```python
from build123d import *

# Parameters (mm, degrees)
SKETCH1_R           = 2.5
BOSS_EXTRUDE1_DEPTH = 9
FILLET1_R           = 0.3
SKETCH2_W           = 3
SKETCH2_H           = 3
CUT_EXTRUDE1_DEPTH  = 4


with BuildPart() as part:
    # Sketch1 → Boss-Extrude1 (new body)
    with BuildSketch(Plane.XY):
        Circle(SKETCH1_R)
    extrude(amount=BOSS_EXTRUDE1_DEPTH)

    # Fillet1
    fillet1_edges = [part.edges().sort_by_distance(p)[0] for p in [
        (-2.5, 0, 9),
    ]]
    fillet(fillet1_edges, radius=FILLET1_R)

    # Sketch2 → Cut-Extrude1 (cut)
    with BuildSketch(Plane(origin=(0, 0, 0), x_dir=(-1, 0, 0), z_dir=(0, 0, -1))):
        Rectangle(SKETCH2_W, SKETCH2_H)
    extrude(amount=-CUT_EXTRUDE1_DEPTH, mode=Mode.SUBTRACT)


solid = part.part
```
Input: part model. Units: mm. Frame: model coordinates. A direction names the side the tool comes from. Round coordinates to 2 decimals unless told otherwise and drop trailing zeros. Loops run counter-clockwise (first coordinate to the right, second up) from the corner with the lowest first, then second, coordinate; pieces in that order, holes last. Notation, with made-up numbers: (20.25, -19.75) - (75.25, -19.75) arc R13 cw to (75.25, -12.75) - close; hole circle Ø7 at (19.25, 37). An arc over 180 degrees is marked (long way). One line per item, written item: value. Start each with the question number.
(1) Section A-A, the plane z = 2.25. Return loops of the section in (x, y).
(2) Access query for faces 5 (the flat face through (0, 0, 9)), 6 (the flat face through (-1.5, 0, 2)). Directions: +Z, -Z, +X, -X, +Y, -Y. A direction counts if a zero-diameter tool reaches every point of the face in a straight line with its end or side. Return the directions, or none.
(3) Section D-D, the plane z = 4.25. Return loops of the section in (x, y), plus the area to 3 significant figures.
(4) Ray query, line 1 (Z direction, x = -0.5, y = -1.2); line 2 (Y direction, x = 0.6, z = 3.5); line 3 (Z direction, x = 0.9, y = 2.05). Return the intervals inside material, ascending. Write a range as [from, to].
(5) Contact query for flat-ended pins moving along their axis: P1, Ø2.5, axis at x = -0.5, y = 0, coming from the -Z side; P2, Ø3, axis at x = -2, z = 5, coming from the +Y side. Output: stop coordinate, or through.
(6) Section B-B, the plane y = 0. Return loops of the section in (x, z).
(7) Draft query along X for faces 1 (the flat face through (2, 0, 0)), 2 (the flat face through (0, -1.5, 2)), 3 (the cylindrical face through (-0.54, -2.44, 4.29)), 4 (the flat face through (0, 1.5, 2)). Return one class per face: +X half, -X half, draft (parallel to the pull), parting line (faces both ways), or undercut.
Results below:
1. outline: circle Ø5 at (0, 0); hole (-1.5, -1.5) - (1.5, -1.5) - (1.5, 1.5) - (-1.5, 1.5) - close
2. face 5: +Z, +X, -X, +Y, -Y
2. face 6: -Z
3. outline: circle Ø5 at (0, 0)
3. area: 19.6 mm^2
4. line 1: [4, 9]
4. line 2: [-2.43, -1.5], [1.5, 2.43]
4. line 3: [0, 9]
5. P1: z = 0
5. P2: y = 2.45
6. outline: (-2.5, 0) - (-1.5, 0) - (-1.5, 4) - (1.5, 4) - (1.5, 0) - (2.5, 0) - (2.5, 8.7) arc R0.3 ccw to (2.2, 9) - (-2.2, 9) arc R0.3 ccw to (-2.5, 8.7) - close
7. face 1: draft
7. face 2: undercut
7. face 3: parting line
7. face 4: undercut
